from build123d import *

# Parameters (mm, degrees)
SKETCH1_W          = 332.4
SKETCH1_H          = 175.4
SKETCH1_R          = 2
BASE_FLANGE1_DEPTH = 0.8
SKETCH2_W          = 221.12
SKETCH2_H          = 130.07
CUT_EXTRUDE1_DEPTH = 10


# Sheet-metal steps are written as plain solids
with BuildPart() as part:
    # Sketch1 → Base-Flange1 (new body)
    with BuildSketch(Plane(origin=(0, 0, 0), x_dir=(1, 0, 0), z_dir=(0, 1, 0))):
        Rectangle(SKETCH1_W, SKETCH1_H)
        with Locations(Location((0, 82.7, 0), (0, 0, 270))):
            Circle(SKETCH1_R, mode=Mode.SUBTRACT)
        with Locations(Location((145, 82.7, 0), (0, 0, 270))):
            Circle(SKETCH1_R, mode=Mode.SUBTRACT)
        with Locations(Location((-145, 82.7, 0), (0, 0, 270))):
            Circle(SKETCH1_R, mode=Mode.SUBTRACT)
        with Locations(Location((-161.2, 36.7, 0), (0, 0, 270))):
            Circle(SKETCH1_R, mode=Mode.SUBTRACT)
        with Locations(Location((161.2, 36.7, 0), (0, 0, 90))):
            Circle(SKETCH1_R, mode=Mode.SUBTRACT)
        with Locations(Location((161.2, -36.7, 0), (0, 0, 270))):
            Circle(SKETCH1_R, mode=Mode.SUBTRACT)
        with Locations(Location((145, -82.7, 0), (0, 0, 90))):
            Circle(SKETCH1_R, mode=Mode.SUBTRACT)
        with Locations(Location((0, -82.7, 0), (0, 0, 90))):
            Circle(SKETCH1_R, mode=Mode.SUBTRACT)
        with Locations(Location((-145, -82.7, 0), (0, 0, 90))):
            Circle(SKETCH1_R, mode=Mode.SUBTRACT)
        with Locations(Location((-161.2, -36.7, 0), (0, 0, 90))):
            Circle(SKETCH1_R, mode=Mode.SUBTRACT)
    extrude(amount=-BASE_FLANGE1_DEPTH)

    # Sketch2 → Cut-Extrude1 (cut)
    with BuildSketch(Plane(origin=(0, 0, 0), x_dir=(1, 0, 0), z_dir=(0, 1, 0))):
        with Locations((-40, 0)):
            Rectangle(SKETCH2_W, SKETCH2_H)
    extrude(amount=-CUT_EXTRUDE1_DEPTH, mode=Mode.SUBTRACT)


solid = part.part
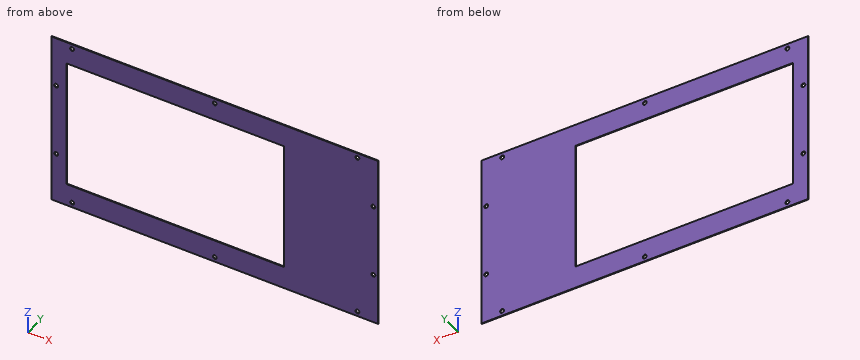
Part model, mm, in its own coordinate system. Coordinates: 2 decimals unless noted, no trailing zeros. Write each loop counter-clockwise with the first axis right and the second up, starting at its lowest first coordinate (ties: lowest second). Pieces come first, ordered by that corner, then holes. Notation, with made-up numbers: (-32.75, 72.5) - (-13.75, 72.5) arc R24 ccw to (-13.75, 110.5) - close; hole circle Ø5 at (-37.5, 70.25). An arc over 180 degrees is marked (long way). Put each result on its own line as item: value.
1. Flat gauge pin, fed straight in: pin 1 Ø3 at (x, z) = (161.2, 36.7) entering from +Y. Where does the tip first touch, or does it go through?
Final values:
pin 1: passes through
2. Band-saw the part on B-B (x = -5.5). Write the cut outline in (y, z) (3 decimals).
Final values:
outline: (-0.8, -87.7) - (0, -87.7) - (0, -65.035) - (-0.8, -65.035) - close; (-0.8, 65.035) - (0, 65.035) - (0, 87.7) - (-0.8, 87.7) - close
3. Probe line 1 along X through (y, z) = (-0.15, 82.7); line 2 along Z through (x, y) = (-145, -0.5) (3 decimals); line 3 along X through (y, z) = (-0.05, 37). List the from-to ranges inside material, lowest first. Write a range as [from, to].
Final values:
line 1: x = [-166.2, -147], [-143, -2], [2, 143], [147, 166.2]
line 2: z = [-87.7, -84.7], [-80.7, -65.035], [65.035, 80.7], [84.7, 87.7]
line 3: x = [-166.2, -163.18], [-159.22, -150.56], [70.56, 159.22], [163.18, 166.2]
4. Band-saw the part on C-C (y = -0.15). Give the number of separate pieces and of enclosed holes in the cut face, then the cut area to 3 significant figures.
Final values:
separate pieces: 1
enclosed holes: 11
area: 29,400 mm²
5. Band-saw the part on A-A (z = 6). Write the cut outline in (x, y), then the cut area to 3 significant figures.
Final values:
outline: (-166.2, -0.8) - (-150.56, -0.8) - (-150.56, 0) - (-166.2, 0) - close; (70.56, -0.8) - (166.2, -0.8) - (166.2, 0) - (70.56, 0) - close
area: 89.0 mm²
